Verification items for the finished model (mm, model axes). A direction names the side the tool comes from. Give positions to 0.01 mm unless a question says otherwise; leave off trailing zeros. Write each loop counter-clockwise with the first axis right and the second up, starting at its lowest first coordinate (ties: lowest second). Pieces come first, ordered by that corner, then holes. Notation, with made-up numbers: (-4, 54.25) - (27, 54.25) arc R12 ccw to (27, 62.25) - close; hole circle Ø10 at (0, 14.25). An arc over 180 degrees is marked (long way). Answer as a JSON object with one key per item and string values. Group by question number.
Item 1: Sectioned sample at B-B, the plane x = -27. Record the boundary of the cut face in (y, z).
Item 2: Draft check along Z on faces 4 (the face through (18.628, 1.014, -1.645)), 5 (the face through (32.5, 1, 4)), 6 (the face through (29.38, 0.99, 12.84)). Enter one of: +Z half, -Z half, draft (parallel to the pull), parting line (faces both ways), or undercut.
Item 3: Tool access check on faces 1 (the face through (16.312, 1.014, 10.547)), 2 (the face through (-18.628, 1.014, -1.645)), 3 (the face through (0, 1, -7)). Record the directions out of +Z, -Z, +X, -X, +Y, -Y that give a thin tool (end or side, any length) a straight path to the whole face; none if there is none.
Item 4: Sectioned sample at A-A, the plane z = 0.8. Record the boundary of the cut face in (x, y).
Item 5: Go/stop test with flat-tipped pins: pin 1 (2 mm diameter, centred on x = -26.5, z = 0.8, fed in from -Y); pin 2 (1 mm diameter, centred on y = 1, z = -4, fed in from -X). Record where each tip stops, or that it passes through.
Item 6: Sectioned sample at D-D, the plane y = 0.6. Record the boundary of the cut face in (x, z).
Item 7: Scan lines: line 1 along X through (y, z) = (1.2, 8.5); line 2 along X through (y, z) = (0.7, 4.25); line 3 along X through (y, z) = (1.4, 8). Record each from-to range of solid material in increasing order. Write a range as [from, to].
Item 8: Sectioned sample at C-C, the plane z = 5.5. Record the boundary of the cut face in (x, y).
```python
from build123d import *

# Parameters (mm, degrees)
SKETCH1_W            = 65
SKETCH1_H            = 14
BOSS_EXTRUDE1_DEPTH  = 2
BOSS_EXTRUDE2_DEPTH  = 2
M3_CLEARANCE_HOLE1_D = 3.4
CUT_EXTRUDE1_DEPTH   = 38.133172501
FILLET1_R            = 7


with BuildPart() as part:
    # Sketch1 → Boss-Extrude1 (new body)
    with BuildSketch(Plane(origin=(0, 0, 0), x_dir=(1, 0, 0), z_dir=(0, 1, 0))):
        Rectangle(SKETCH1_W, SKETCH1_H)
    extrude(amount=BOSS_EXTRUDE1_DEPTH)

    # Sketch5 → Boss-Extrude2 (add)
    with BuildSketch(Plane(origin=(0, 2, 0), x_dir=(1, 0, 0), z_dir=(0, 1, 0))):
        Polygon((-32.5, -7), (-32.5, -17.85), (-8.45, -7), align=None)
        Polygon((8.45, -7), (32.5, -7), (32.5, -17.85), align=None)
    extrude(amount=-BOSS_EXTRUDE2_DEPTH)

    # M3 Clearance Hole1 (through all)
    with Locations(Plane(origin=(0, 2, 0), x_dir=(1, 0, 0), z_dir=(0, 1, 0))):
        with Locations((-26.5, -0.8), (26.5, -0.8)):
            Hole(M3_CLEARANCE_HOLE1_D / 2)

    # Sketch4 → Cut-Extrude1 (cut, through all)
    with BuildSketch(Plane(origin=(0, 2, 0), x_dir=(1, 0, 0), z_dir=(0, 1, 0))):
        with BuildLine():
            ThreePointArc((-24.14980848, -10.200572933), (-18.574782967, -6.375401925), (-16.858188636, 0.164181136))
            ThreePointArc((-16.858188636, 0.164181136), (-18.664181136, 1.641811364), (-20.141811364, -0.164181136))
            ThreePointArc((-20.141811364, -0.164181136), (-21.273800865, -4.476638541), (-24.950191053, -6.999106435))
            ThreePointArc((-24.950191053, -6.999106435), (-26.150733249, -9.000031029), (-24.14980848, -10.200572933))
        make_face()
        with BuildLine():
            ThreePointArc((24.14980848, -10.200572933), (18.574782967, -6.375401925), (16.858188636, 0.164181136))
            ThreePointArc((16.858188636, 0.164181136), (18.664181136, 1.641811364), (20.141811364, -0.164181136))
            ThreePointArc((20.141811364, -0.164181136), (21.273800865, -4.476638541), (24.950191053, -6.999106435))
            ThreePointArc((24.950191053, -6.999106435), (26.150733249, -9.000031029), (24.14980848, -10.200572933))
        make_face()
    extrude(amount=-CUT_EXTRUDE1_DEPTH, mode=Mode.SUBTRACT)

    # Fillet1
    fillet1_edges = [part.edges().sort_by_distance(p)[0] for p in [
        (32.5, 1, -7),
        (-32.5, 1, -7),
        (32.5, 1, 17.85),
        (8.45, 1, 7),
        (-8.45, 1, 7),
        (-32.5, 1, 17.85),
    ]]
    fillet(fillet1_edges, radius=FILLET1_R)


solid = part.part
```
Geometry check:
{
 "1": {"outline": "(0, -6.84) - (2, -6.84) - (2, -0.82) - (0, -0.82) - close; (0, 2.42) - (2, 2.42) - (2, 13.85) - (0, 13.85) - close"},
 "2": {"face 4": "undercut", "face 5": "draft", "face 6": "+Z half"},
 "3": {"face 1": "+Z, +Y, -Y", "face 2": "+Y, -Y", "face 3": "-Z, +X, -X, +Y, -Y"},
 "4": {"outline": "(-32.5, 0) - (-28.2, 0) - (-28.2, 2) - (-32.5, 2) - close; (-24.8, 0) - (-20.11, 0) - (-20.11, 2) - (-24.8, 2) - close; (-16.81, 0) - (16.81, 0) - (16.81, 2) - (-16.81, 2) - close; (20.11, 0) - (24.8, 0) - (24.8, 2) - (20.11, 2) - close; (28.2, 0) - (32.5, 0) - (32.5, 2) - (28.2, 2) - close"},
 "5": {"pin 1": "through", "pin 2": "x = -31.56"},
 "6": {"outline": "(-32.5, 0) arc R7 ccw to (-25.5, -7) - (25.5, -7) arc R7 ccw to (32.5, 0) - (32.5, 7.01) arc R7 ccw to (22.62, 13.39) - (9.82, 7.62) arc R7 cw to (6.94, 7) - (-6.94, 7) arc R7 cw to (-9.82, 7.62) - (-22.62, 13.39) arc R7 ccw to (-32.5, 7.01) - close; hole circle Ø3.4 at (-26.5, 0.8); hole (-24.95, 7) arc R6.39 cw to (-20.14, 0.16) arc R1.65 ccw to (-16.86, -0.16) arc R9.69 ccw to (-24.15, 10.2) arc R1.65 ccw to start; hole (16.86, -0.16) arc R1.65 ccw to (20.14, 0.16) arc R6.39 cw to (24.95, 7) arc R1.65 ccw to (24.15, 10.2) arc R9.69 ccw to start; hole circle Ø3.4 at (26.5, 0.8)"},
 "7": {"line 1": "[-32.34, -26.2], [-20.62, -11.77], [11.77, 20.62], [26.2, 32.34]", "line 2": "[-32.5, -21.12], [-17.45, 17.45], [21.12, 32.5]", "line 3": "[-32.43, -26.09], [-20.02, -10.67], [10.67, 20.02], [26.09, 32.43]"},
 "8": {"outline": "(-32.5, 0) - (-22.17, 0) - (-22.17, 2) - (-32.5, 2) - close; (-18.03, 0) - (18.03, 0) - (18.03, 2) - (-18.03, 2) - close; (22.17, 0) - (32.5, 0) - (32.5, 2) - (22.17, 2) - close"}
}
